Autodesk Fusion 360 part; units mm, degrees
sketch "ratchet scketch & pawl" plane through (0, 0, 0) normal (0, 1, 0) x (1, 0, 0)
  circle A0 centre (0, 0) radius 7.75 construction
  circle A1 centre (0, 0) radius 6.5 construction
  line L0 (0, 0) -> (1.3458, 7.6323) construction
  line L1 (0, 0) -> (-2.8494, 5.8422) construction
  arc A2 (1.3458, 7.6323) -> (-2.8494, 5.8422) centre (0.5379, 3.7147) ccw construction
  line L2 (0, 0) -> (6.5, 0) construction
  line L3 (0, 0) -> (4.4082, 25) construction
  circle A3 centre (2.9976, 17) radius 1.5
  circle A4 centre (2.9976, 17) radius 2.5
  line L4 (-2.8494, 5.8422) -> (-0.2045, 20.8422) construction
  line L5 (-2.8494, 5.8422) -> (-3.5335, 7.7215)
  arc A5 (4.0328, 14.7244) -> (-2.8494, 5.8422) centre (9.0259, 3.7482) ccw
  arc A6 (2.2215, 19.3765) -> (-3.5335, 7.7215) centre (5.0435, 10.7347) ccw
  circle A7 centre (-2.6702, 10.3422) radius 1.25
  dimension "d28" = 13
  dimension "d29" = 15.5
  dimension "d30" = 80
  dimension "d31" = 36
  dimension "d32" = 4
  dimension "d33" = 25
  dimension "d34" = 3
  dimension "d35" = 5
  dimension "d36" = 15
  dimension "d37" = 2
  dimension "d40" = 30
  dimension "d43" = 9.0909
  dimension "d44" = 17
  dimension "d45" = 2.5
  dimension "d46" = 4.5
  dimension "d47" = 7.7237
extrude "Extrude1" add sketch "ratchet scketch & pawl" along normal blind 5 contours A4 | A4 L5 A5 A6 | A7 makes body 1
move_body "Move1" bodies 1 to x (0, 0, 1) y (0, 1, 0) z (-1, 0, 0) at (-3.7668, 0, 14.8212)
extrude "Extrude2" add sketch "ratchet scketch & pawl" along normal blind 5 separate body contours A4 | A4 L5 A5 A6 | A7 makes body 2
extrude "Extrude3" add sketch "ratchet scketch & pawl" along normal blind 5 from surface at 5 contours A7 bodies 2
delete_body "RemoveBody1" bodies 1
equation "d29 = ( 7.75 * 2 ) * 1 mm"
The listing builds one solid part. Answer for the finished solid, in the listing's coordinates (mm). Coordinates: 2 decimals unless noted, no trailing zeros. Loops run counter-clockwise (first coordinate to the right, second up) from the corner with the lowest first, then second, coordinate; pieces in that order, holes last. Notation, with made-up numbers: (21, 7) -> (51, 7) arc R17 cw to (51, 25) -> close; hole circle Ø4 at (-32.75, -20). An arc over 180 degrees is marked (long way). Return JSON: item names as keys, results as strings. Group by question number.
(1) Find the intervals of material crossed by probe 1 along X at (y, z) = (3.35, -17); probe 2 along Y at (x, z) = (1, -17); probe 3 along X at (y, z) = (4.25, -16.75), in increasing order. Write a range as from..to.
(2) A cutting plane is placed at B-B on y = 4.5. Write down the section's boundary in (x, z), and give its area (3 significant figures).
(3) A cutting plane is placed at C-C on z = -17. Write down the section's boundary in (x, y), and give its area (3 significant figures).
(4) A cutting plane is placed at D-D on x = -1.75. Write down the section's boundary in (y, z).
(5) A cutting plane is placed at A-A on x = 2.75. Write down the section's boundary in (y, z), and give its area (3 significant figures).
(6) Determine the mould class of faces 1 (the cylindrical face through (-1.478, 7.465, -9.967)), 2 (the cylindrical face through (-0.556, 2.465, -11.069)), 3 (the cylindrical face through (3.804, 2.465, -15.735)) for opening direction X: released by +X, released by -X, zero draft, split by the parting line, or undercut.
(7) Given pin 1 Ø4 at (x, z) = (-1.5, -14) entering from -Y; pin 2 Ø5 at (x, z) = (-1.5, -16.5) entering from +Y; pin 3 Ø2 at (x, y) = (0.5, 3.5) entering from -Z; pin 4 Ø6 at (y, z) = (2, -13.5) entering from +X, each flat-ended and moving along its own axis, determine where each tip first touches the part or whether it passes through.
The answers:
{
 "1": {"probe 1": "x = -1.54..1.5, 4.5..5.5", "probe 2": "y = 0..5", "probe 3": "x = -1.77..1.52, 4.48..5.49"},
 "2": {"outline": "(-3.53, -7.72) arc R9.09 ccw to (2.22, -19.38) arc R2.5 ccw to (4.03, -14.72) arc R12.06 cw to (-2.85, -5.84) -> close; hole circle Ø3 at (3, -17)", "area": "49.5 mm^2"},
 "3": {"outline": "(-1.54, 0) -> (1.5, 0) -> (1.5, 5) -> (-1.54, 5) -> close; (4.5, 0) -> (5.5, 0) -> (5.5, 5) -> (4.5, 5) -> close", "area": "20.2 mm^2"},
 "4": {"outline": "(0, -16.78) -> (5, -16.78) -> (5, -11.19) -> (10, -11.19) -> (10, -9.5) -> (5, -9.5) -> (5, -9.16) -> (0, -9.16) -> close"},
 "5": {"outline": "(0, -19.49) -> (5, -19.49) -> (5, -18.48) -> (0, -18.48) -> close; (0, -15.52) -> (5, -15.52) -> (5, -14.04) -> (0, -14.04) -> close", "area": "12.4 mm^2"},
 "6": {"face 1": "split by the parting line", "face 2": "released by +X", "face 3": "undercut"},
 "7": {"pin 1": "stops at y = 0", "pin 2": "stops at y = 5", "pin 3": "stops at z = -19.11", "pin 4": "stops at x = 5.45"}
}
